from build123d import *

# Parameters (mm, degrees)
F3_R     = 8.8335869627
F4_DEPTH = 558.8
F5_SIZE  = 7.62
F6_ANGLE = 90


with BuildPart() as f1:
    # F0 (on Right) → F1 (revolve)
    with BuildSketch(Plane.YZ):
        with BuildLine():
            Line((0, -19.05), (0, 0))
            Line((0, 0), (0, 19.05))
            Line((0, 19.05), (-19.05, 19.05))
            ThreePointArc((-19.05, 19.05), (-10.4505208253, 0), (-19.05, -19.05))
            Line((-19.05, -19.05), (0, -19.05))
        make_face()
    revolve(axis=Axis((0, -35.8505208253, 12.1182259172), (0, 0, 1)))

    # F3 (on offset) → F4 (join)
    with BuildSketch(Plane.XZ.offset(7.62)):
        Circle(F3_R)
    extrude(amount=-F4_DEPTH)

    # F5
    f5_edges = [f1.edges().sort_by_distance(p)[0] for p in [
        (0, -71.701042, 19.05),
        (0, -71.701042, -19.05),
    ]]
    chamfer(f5_edges, length=F5_SIZE)


with BuildPart() as f1_1:
    # F6: moved
    add(f1.part.rotate(Axis((0, -7.62, 0), (0, -1, 0)), F6_ANGLE))


solid = f1_1.part
The model under review builds one solid part; all positions refer to its coordinate system, in mm. A direction names the side the tool comes from. Round coordinates to 2 decimals unless told otherwise and drop trailing zeros. Order: outer loops, then holes, each group sorted by start corner. A loop starts at its lowest first (then second) coordinate and runs counter-clockwise, first axis right, second up. Notation, with made-up numbers: (-1.5, 57.25) -> (7.5, 57.25) arc R13 cw to (7.5, 67.25) -> close; hole circle Ø2 at (82.25, 87). An arc over 180 degrees is marked (long way). Use CSV: the item, a comma, the result in double quotes. Start each with the question number.
(1) Wall thickness on probe 1 along Z at (x, y) = (1, 461); probe 2 along Z at (x, y) = (-10.5, -30.5): over which ranges is each line inside the solid? List them lowest first. Write a range as from..to.
(2) Tool access review of faces 1 (the face through (18.68, -8.57, -8.59)), 2 (the face through (-2.653, 271.171, 8.426)): name each direction out of +Z, -Z, +X, -X, +Y, -Y from which nothing blocks a thin tool from reaching the whole face with its end or side.
(3) Mouldability with a two-part tool opening along Y and no side actions: class faces 3 (the face through (19.05, -48, 12)), 4 (the face through (-18.68, -8.57, -8.59)), 5 (the face through (0, 551.18, 0)) as pulls with the +Y half, pulls with the -Y half, needs draft (parallel to the pull), parting line crosses it, or undercut.
(4) Consider section B-B on z = 0. Write out the cut boundary in (x, y).
(5) Insertion check: pin 1 (10 mm diameter, centred on x = -6, y = 422.5, fed in from +Z); pin 2 (8 mm diameter, centred on y = 157, z = -0.5, fed in from +X); pin 3 (5 mm diameter, centred on x = 5, y = 189.5, fed in from +Z). Each pin has a flat end and moves straight along its axis. Give the tip position at first contact, or say it passes through.
(6) Consider section C-C on y = 256.5. Write out the cut boundary in (x, z), and give its area (3 significant figures).
(7) Consider section A-A on x = 0. Write out the cut boundary in (y, z), and give its area (3 significant figures).
Responses:
1,probe 1,"-8.78..8.78"
1,probe 2,"-35.45..-22.5, 22.5..35.45"
2,face 1,"+X"
2,face 2,"+Y"
3,face 3,"needs draft"
3,face 4,"parting line crosses it"
3,face 5,"pulls with the +Y half"
4,outline,"(-19.05, -64.08) -> (-11.43, -71.7) -> (11.43, -71.7) -> (19.05, -64.08) -> (19.05, -52.65) arc R25.4 cw to (-19.05, -52.65) -> close; (-19.05, -19.05) arc R25.4 cw to (19.05, -19.05) -> (19.05, -7.62) -> (11.43, 0) -> (8.83, 0) -> (8.83, 551.18) -> (-8.83, 551.18) -> (-8.83, 0) -> (-11.43, 0) -> (-19.05, -7.62) -> close"
5,pin 1,"z = 8.78"
5,pin 2,"x = 8.83"
5,pin 3,"z = 8.47"
6,outline,"circle Ø17.67 at (0, 0)"
6,area,"245 mm²"
7,outline,"(-1.11, -8.83) -> (551.18, -8.83) -> (551.18, 8.83) -> (-1.11, 8.83) arc R35.85 ccw (long way) to start; hole circle Ø50.8 at (-35.85, 0)"
7,area,"11,800 mm²"
